from build123d import *

# Parameters (mm, degrees)
F0_W     = 95
F0_H     = 50
F1_DEPTH = 30
F2_R     = 10
F3_DEPTH = 10


with BuildPart() as f1:
    # F0 (on Top) → F1 (new body)
    with BuildSketch(Plane.XY):
        with Locations((47.5, 0)):
            Rectangle(F0_W, F0_H)
    extrude(amount=F1_DEPTH)

    # F2 (on face) → F3 (cut)
    with BuildSketch(Plane.XY.offset(30)):
        with Locations((15, 0)):
            Circle(F2_R)
        with Locations((45, 0)):
            Circle(F2_R)
        with Locations((75, 0)):
            Circle(F2_R)
    extrude(amount=-F3_DEPTH, mode=Mode.SUBTRACT)

    # F4: F1 across face


with BuildPart() as f1_1:
    add(f1.part)
    add(f1.part.mirror(Plane(origin=(0, 0, 15), x_dir=(0, -1, 0), z_dir=(-1, 0, 0))))


solid = f1_1.part
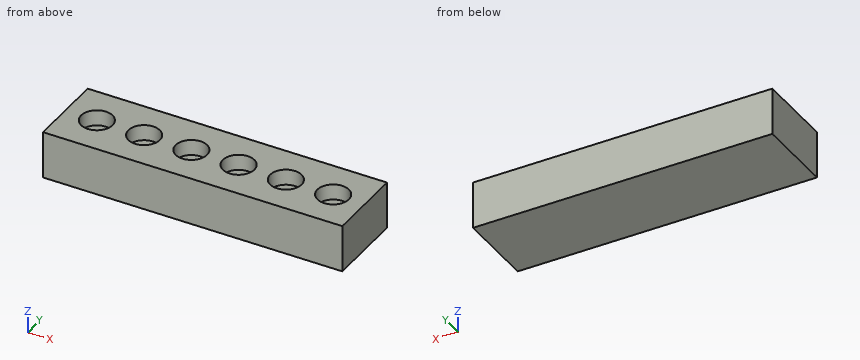
The listing builds one solid part. Answer for the finished solid, in the listing's coordinates (mm). Give positions to 0.01 mm unless a question says otherwise; leave off trailing zeros. Write each loop counter-clockwise with the first axis right and the second up, starting at its lowest first coordinate (ties: lowest second). Pieces come first, ordered by that corner, then holes.
1) Find the intervals of material crossed by L1, parallel to Y at x = -45, z = 27.25; L2, parallel to Y at x = 78, z = 24.5; L3, parallel to Z at x = -11, y = -7.5, in increasing order.
2) Section A-A (x = 81.5) is taken. Write down the section's boundary in (y, z), and give its area (3 significant figures).
3) Section B-B (y = -3.5) is taken. Write down the section's boundary in (x, z).
4) Section C-C (x = 45) is taken. Write down the section's boundary in (y, z).
5) Given P1, Ø16, axis at x = 75, y = 0, coming from the +Z side, flat-ended and moving along its own axis, determine where the tip first touches the part or whether it passes through.
Response:
1. L1: y = -25 to -10, 10 to 25
1. L2: y = -25 to -9.54, 9.54 to 25
1. L3: z = 0 to 20
2. outline: (-25, 0) - (25, 0) - (25, 30) - (7.6, 30) - (7.6, 20) - (-7.6, 20) - (-7.6, 30) - (-25, 30) - close
2. area: 1,350 mm2
3. outline: (-95, 0) - (95, 0) - (95, 30) - (84.37, 30) - (84.37, 20) - (65.63, 20) - (65.63, 30) - (54.37, 30) - (54.37, 20) - (35.63, 20) - (35.63, 30) - (24.37, 30) - (24.37, 20) - (5.63, 20) - (5.63, 30) - (-5.63, 30) - (-5.63, 20) - (-24.37, 20) - (-24.37, 30) - (-35.63, 30) - (-35.63, 20) - (-54.37, 20) - (-54.37, 30) - (-65.63, 30) - (-65.63, 20) - (-84.37, 20) - (-84.37, 30) - (-95, 30) - close
4. outline: (-25, 0) - (25, 0) - (25, 30) - (10, 30) - (10, 20) - (-10, 20) - (-10, 30) - (-25, 30) - close
5. P1: stops at z = 20
